```python
from build123d import *

# Parameters (mm, degrees)
SKETCH_1_W           = 150
SKETCH_1_H           = 160
EXTRUDE_1_DEPTH      = 30
FILLET_1_R           = 5
SKETCH_3_W           = 140
SKETCH_3_H           = 152
CUT_EXTRUDE_2_DEPTH  = 26
SKETCH_9_W           = 6
SKETCH_9_H           = 3
CUT_EXTRUDE_7_DEPTH  = 151
FILLET_2_R           = 2
SKETCH_11_R          = 1.65
CUT_EXTRUDE_8_DEPTH  = 8
SKETCH_12_W          = 6.5
SKETCH_12_H          = 3.3
CUT_EXTRUDE_9_DEPTH  = 15
SKETCH_16_W          = 35
SKETCH_16_H          = 20
CUT_EXTRUDE_12_DEPTH = 40
SKETCH_17_R          = 1.65
CUT_EXTRUDE_13_DEPTH = 10


with BuildPart() as part:
    # 草图1 → 凸台-拉伸1 (new body)
    with BuildSketch(Plane(origin=(0, 0, 0), x_dir=(1, 0, 0), z_dir=(0, 1, 0))):
        Rectangle(SKETCH_1_W, SKETCH_1_H)
    extrude(amount=EXTRUDE_1_DEPTH)

    # 圆角1
    fillet_1_edges = [part.edges().sort_by_distance(p)[0] for p in [
        (75, 15, 80),
        (-75, 15, 80),
        (-75, 15, -80),
        (75, 15, -80),
    ]]
    fillet(fillet_1_edges, radius=FILLET_1_R)

    # 草图3 → 切除-拉伸2 (cut)
    with BuildSketch(Plane.XZ):
        Rectangle(SKETCH_3_W, SKETCH_3_H)
    extrude(amount=-CUT_EXTRUDE_2_DEPTH, mode=Mode.SUBTRACT)

    # 草图9 → 切除-拉伸7 (cut, through all)
    with BuildSketch(Plane.ZY.offset(75)):
        with Locations((65, 24.5)):
            Rectangle(SKETCH_9_W, SKETCH_9_H)
        with Locations((-15, 24.5)):
            Rectangle(SKETCH_9_W, SKETCH_9_H)
    extrude(amount=-CUT_EXTRUDE_7_DEPTH, mode=Mode.SUBTRACT)

    # 圆角2
    fillet_2_edges = [part.edges().sort_by_distance(p)[0] for p in [
        (-70, 13, -76),
        (-70, 13, 76),
        (70, 13, 76),
        (70, 13, -76),
    ]]
    fillet(fillet_2_edges, radius=FILLET_2_R)

    # 草图11 → 切除-拉伸8 (cut)
    with BuildSketch(Plane(origin=(0, 30, 0), x_dir=(1, 0, 0), z_dir=(0, 1, 0))):
        with Locations((0, 76)):
            Circle(SKETCH_11_R)
    extrude(amount=-CUT_EXTRUDE_8_DEPTH, mode=Mode.SUBTRACT)

    # 草图12 → 切除-拉伸9 (cut)
    with BuildSketch(Plane(origin=(0, 0, -80), x_dir=(-1, 0, 0), z_dir=(0, 0, -1))):
        with Locations((0, 23.35)):
            Rectangle(SKETCH_12_W, SKETCH_12_H)
    extrude(amount=-CUT_EXTRUDE_9_DEPTH, mode=Mode.SUBTRACT)

    # 草图16 → 切除-拉伸12 (cut)
    with BuildSketch(Plane.XY.offset(80)):
        with Locations((37.995108753, 14.88178475)):
            Rectangle(SKETCH_16_W, SKETCH_16_H)
        with Locations((-37.995108753, 14.88178475)):
            Rectangle(SKETCH_16_W, SKETCH_16_H)
    extrude(amount=-CUT_EXTRUDE_12_DEPTH, mode=Mode.SUBTRACT)

    # 草图17 → 切除-拉伸13 (cut)
    with BuildSketch(Plane(origin=(0, 30, 0), x_dir=(1, 0, 0), z_dir=(0, 1, 0))):
        with Locations((-72.6, -65)):
            Circle(SKETCH_17_R)
        with Locations((72.6, -65)):
            Circle(SKETCH_17_R)
        with Locations((-72.6, 15)):
            Circle(SKETCH_17_R)
        with Locations((72.6, 15)):
            Circle(SKETCH_17_R)
    extrude(amount=-CUT_EXTRUDE_13_DEPTH, mode=Mode.SUBTRACT)


solid = part.part
```
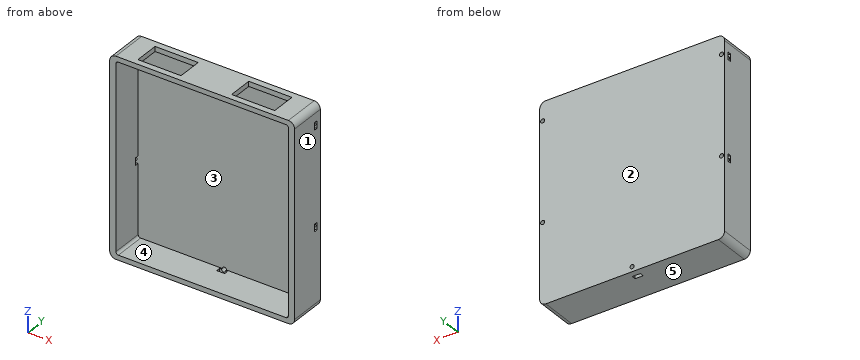
For this review, take the finished solid that the model builds, in its own axes (mm). Face numbers are marked on the shaded views. A direction names the side the tool comes from. Coordinates: 2 decimals unless noted, no trailing zeros. Loops run counter-clockwise (first coordinate to the right, second up) from the corner with the lowest first, then second, coordinate; pieces in that order, holes last.
1. Add section D-D, the plane z = -62. Give the boundary of the cut face in (x, y), then the cut area to 3 significant figures.
2. Add section C-C, the plane x = 14.5. Give the boundary of the cut face in (y, z).
3. Mouldability with a two-part tool opening along X and no side actions: class the marked faces 1, 2 and 3 as +X half, -X half, draft (parallel to the pull), parting line (faces both ways), or undercut.
4. For line 1 (X direction, y = 20.8, z = -15); line 2 (X direction, y = 12, z = 50); line 3 (X direction, y = 28.8, z = 65), list the stretches that pass through material, from the lowest coordinate up.
5. Add section A-A, the plane y = 17. Give the boundary of the cut face in (x, z).
6. For the marked faces 4 and 5, list the 3-axis set-ups (+Z, -Z, +X, -X, +Y, -Y) from which the entire face can be reached by the end or side of a thin tool; tool diameter is ignored.
7. Insertion check: P1, Ø3.5, axis at y = 24, z = -79, coming from the -X side; P2, Ø2, axis at y = 12, z = 77.5, coming from the -X side; P3, Ø8, axis at x = -27, y = 19.5, coming from the +Z side. Each pin has a flat end and moves straight along its axis. Give the tip position at first contact, or say it passes through.
8. Add section B-B, the plane x = 31.5. Give the boundary of the cut face in (y, z), then the cut area to 3 significant figures.
Result:
1. outline: (-75, 0) - (-70, 0) - (-70, 26) - (70, 26) - (70, 0) - (75, 0) - (75, 30) - (-75, 30) - close
1. area: 860 mm2
2. outline: (0, -80) - (30, -80) - (30, 80) - (0, 80) - (0, 76) - (26, 76) - (26, -76) - (0, -76) - close
3. face 1: +X half
3. face 2: draft
3. face 3: undercut
4. line 1: x = -75 to -74.25, -70.95 to -70, 70 to 70.95, 74.25 to 75
4. line 2: x = -75 to -70, 70 to 75
4. line 3: x = -75 to -74.25, -70.95 to 70.95, 74.25 to 75
5. outline: (-75, -75) arc R5 ccw to (-70, -80) - (70, -80) arc R5 ccw to (75, -75) - (75, 75) arc R5 ccw to (70, 80) - (55.5, 80) - (55.5, 76) - (68, 76) arc R2 cw to (70, 74) - (70, -74) arc R2 cw to (68, -76) - (-68, -76) arc R2 cw to (-70, -74) - (-70, 74) arc R2 cw to (-68, 76) - (-55.5, 76) - (-55.5, 80) - (-70, 80) arc R5 ccw to (-75, 75) - close; (-20.5, 76) - (20.5, 76) - (20.5, 80) - (-20.5, 80) - close
6. face 4: -Y
6. face 5: -Z, +X, -X, +Y, -Y
7. P1: stops at x = -74.47
7. P2: stops at x = -74.77
7. P3: stops at z = -76
8. outline: (0, -80) - (30, -80) - (30, 80) - (24.88, 80) - (24.88, 76) - (26, 76) - (26, -76) - (0, -76) - close; (0, 76) - (4.88, 76) - (4.88, 80) - (0, 80) - close
8. area: 768 mm2
